```python
from build123d import *

# Parameters (mm, degrees)
F0_R      = 12.5
F1_DEPTH  = 22
F2_R      = 12.2
F3_DEPTH  = 30.8
F4_R      = 3.5
F5_DEPTH  = 2.5
F6_R      = 2
F7_DEPTH  = 12.5
F9_DEPTH  = 8
F10_R     = 1.5
F11_DEPTH = 4


with BuildPart() as f1:
    # F0 (on Top) → F1 (new body)
    with BuildSketch(Plane.XY):
        Circle(F0_R)
    extrude(amount=-F1_DEPTH)

    # F2 (on face) → F3 (join)
    with BuildSketch(Plane(origin=(0, 0, -22), x_dir=(1, 0, 0), z_dir=(0, 0, -1))):
        Circle(F2_R)
    extrude(amount=F3_DEPTH)

    # F4 (on face) → F5 (join)
    with BuildSketch(Plane.XY):
        Circle(F4_R)
    extrude(amount=F5_DEPTH)

    # F6 (on face) → F7 (join)
    with BuildSketch(Plane.XY):
        Circle(F6_R)
    extrude(amount=F7_DEPTH)

    # F8 (on face) → F9 (cut)
    with BuildSketch(Plane.XY.offset(12.5)):
        with BuildLine():
            Line((1.322876, -1.5), (-1.322876, -1.5))
            ThreePointArc((-1.322876, -1.5), (0, -2), (1.322876, -1.5))
        make_face()
    extrude(amount=-F9_DEPTH, mode=Mode.SUBTRACT)

    # F10 (on face) → F11 (cut)
    with BuildSketch(Plane.XY):
        with Locations((-8.5, 0)):
            Circle(F10_R)
        with Locations((8.5, 0)):
            Circle(F10_R)
    extrude(amount=-F11_DEPTH, mode=Mode.SUBTRACT)


solid = f1.part
```
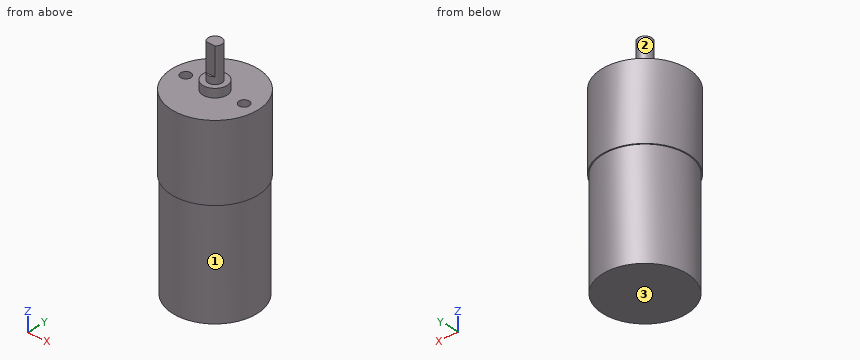
Geometry: final body of the model. Coordinates: model frame, mm. Face numbers are marked on the shaded views. A direction names the side the tool comes from. Round coordinates to 2 decimals unless told otherwise and drop trailing zeros. Write each loop counter-clockwise with the first axis right and the second up, starting at its lowest first coordinate (ties: lowest second). Pieces come first, ordered by that corner, then holes. Notation, with made-up numbers: (-14, 8) -> (29, 8) arc R19 ccw to (29, 20) -> close; hole circle Ø5 at (-22.5, -33.5). An arc over 180 degrees is marked (long way). Use CSV: the item, a comma, the result in double quotes. Start each with the question number.
Q1. Line query: L1, parallel to Z at x = -0.75, y = 4.75; L2, parallel to Z at x = -0.5, y = -3.25; L3, parallel to Y at x = 8.5, z = -2.45. Output: solid intervals per line, ascending.
Q2. First-contact query: pin 1 Ø3.5 at (x, y) = (-8.5, 0.5) entering from +Z; pin 2 Ø4 at (x, z) = (-2, -21) entering from -Y; pin 3 Ø1.3 at (x, z) = (0.5, 9) entering from -Y; pin 4 Ø1.5 at (y, z) = (-5.5, -41.5) entering from -X. Flat tips, straight axial feed; report the tip coordinate or a pass-through.
Q3. Section D-D (x = -6). Return loops of the section in (y, z), plus the area to 3 significant figures.
Q4. Reachability of the marked faces 1, 2 and 3 from +Z, -Z, +X, -X, +Y, -Y: full face, straight path, thin tool, end or side. Return the list, or none.
Q5. Section A-A (x = 0). Return loops of the section in (y, z).
Q6. Section B-B (y = -9.25). Return loops of the section in (x, z), plus the area to 3 significant figures.
Q7. Section C-C (z = -44). Return loops of the section in (x, y).
Result sheet:
1,L1,"-52.8 to 0"
1,L2,"-52.8 to 2.5"
1,L3,"-9.17 to -1.5, 1.5 to 9.17"
2,pin 1,"z = 0"
2,pin 2,"y = -12.5"
2,pin 3,"y = -1.5"
2,pin 4,"x = -11.24"
3,outline,"(-10.97, -22) -> (-10.62, -22) -> (-10.62, -52.8) -> (10.62, -52.8) -> (10.62, -22) -> (10.97, -22) -> (10.97, 0) -> (-10.97, 0) -> close"
3,area,"1,140 mm²"
4,face 1,"-Z"
4,face 2,"+Z"
4,face 3,"-Z, +X, -X, +Y, -Y"
5,outline,"(-12.5, -22) -> (-12.2, -22) -> (-12.2, -52.8) -> (12.2, -52.8) -> (12.2, -22) -> (12.5, -22) -> (12.5, 0) -> (3.5, 0) -> (3.5, 2.5) -> (2, 2.5) -> (2, 12.5) -> (-1.5, 12.5) -> (-1.5, 4.5) -> (-2, 4.5) -> (-2, 2.5) -> (-3.5, 2.5) -> (-3.5, 0) -> (-12.5, 0) -> close"
6,outline,"(-8.41, -22) -> (-7.95, -22) -> (-7.95, -52.8) -> (7.95, -52.8) -> (7.95, -22) -> (8.41, -22) -> (8.41, 0) -> (-8.41, 0) -> close"
6,area,"860 mm²"
7,outline,"circle Ø24.4 at (0, 0)"
